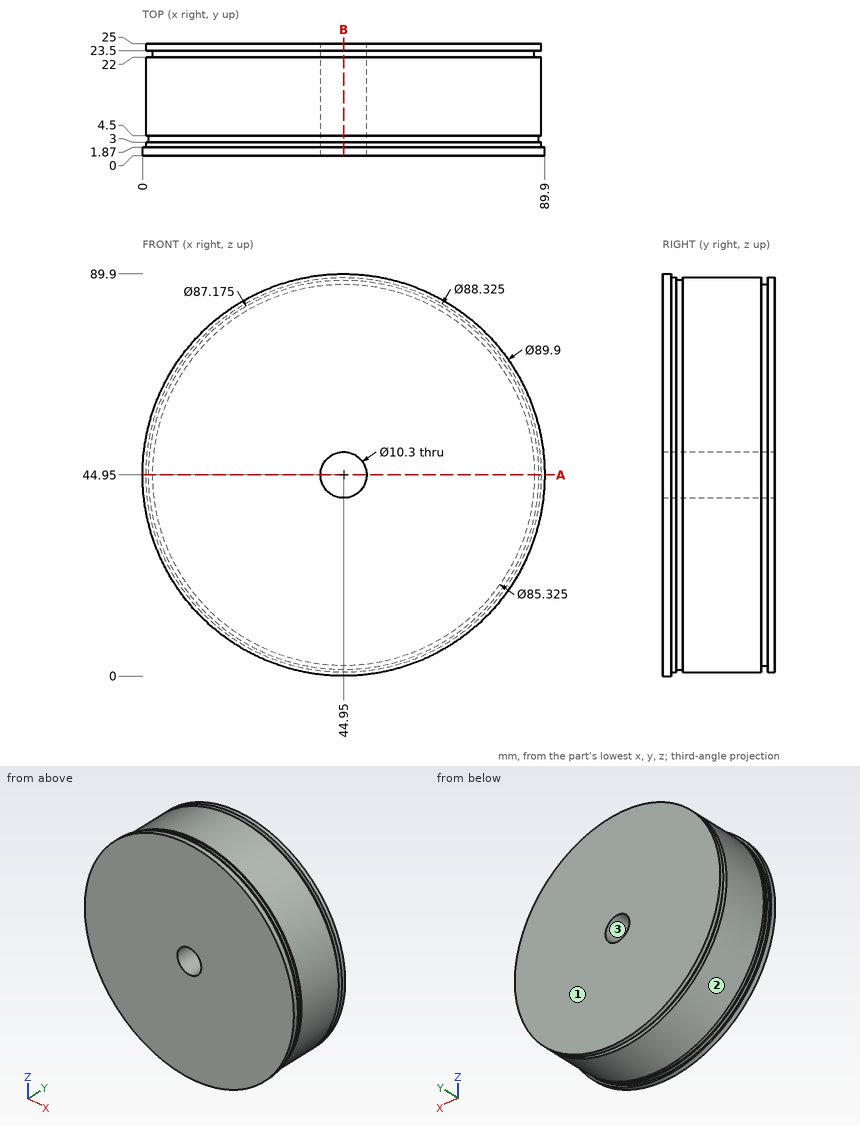
Design review of the part shown in the three views and the two pictorial views. Dimensions are in mm from the part's minimum x, y and z. Round coordinates to 2 decimals unless told otherwise and drop trailing zeros. Order: outer loops, then holes, each group sorted by start corner. A loop starts at its lowest first (then second) coordinate and runs counter-clockwise, first axis right, second up.
(1) Mouldability with a two-part tool opening along X and no side actions: class the marked faces 1, 2 and 3 as released by +X, released by -X, zero draft, split by the parting line, or undercut.
Working result:
face 1: zero draft
face 2: split by the parting line
face 3: undercut
(2) Wall thickness on L1, parallel to Y at x = 7, z = 67; L2, parallel to Z at x = 44.95, y = 17; L3, parallel to X at y = 19.5, z = 38: over which ranges is each line inside the solid? List them lowest first.
Working result:
L1: y = 0 to 3, 4.5 to 22, 23.5 to 25
L2: z = 0.79 to 39.8, 50.1 to 89.11
L3: x = 1.34 to 88.56
(3) Take a section at B-B, the plane x = 44.95. State the section outline as (y, z) points.
Working result:
outline: (0, 0) - (1.87, 0) - (1.87, 0.79) - (3, 0.79) - (3, 1.36) - (4.5, 1.36) - (4.5, 0.79) - (22, 0.79) - (22, 2.29) - (23.5, 2.29) - (23.5, 0.79) - (25, 0.79) - (25, 39.8) - (0, 39.8) - close; (0, 50.1) - (25, 50.1) - (25, 89.11) - (23.5, 89.11) - (23.5, 87.61) - (22, 87.61) - (22, 89.11) - (4.5, 89.11) - (4.5, 88.54) - (3, 88.54) - (3, 89.11) - (1.87, 89.11) - (1.87, 89.9) - (0, 89.9) - close
(4) Take a section at A-A, the plane z = 44.95. State the section outline as (x, y) points.
Working result:
outline: (0, 0) - (39.8, 0) - (39.8, 25) - (0.79, 25) - (0.79, 23.5) - (2.29, 23.5) - (2.29, 22) - (0.79, 22) - (0.79, 4.5) - (1.36, 4.5) - (1.36, 3) - (0.79, 3) - (0.79, 1.87) - (0, 1.87) - close; (50.1, 0) - (89.9, 0) - (89.9, 1.87) - (89.11, 1.87) - (89.11, 3) - (88.54, 3) - (88.54, 4.5) - (89.11, 4.5) - (89.11, 22) - (87.61, 22) - (87.61, 23.5) - (89.11, 23.5) - (89.11, 25) - (50.1, 25) - close
(5) For P1, Ø6, axis at y = 22.5, z = 50.5, coming from the +X side; P2, Ø10, axis at x = 73, y = 14.5, coming from the -Z side; P3, Ø10, axis at y = 3, z = 18, coming from the -X side, all flat-tipped, find the tip position at first contact; note any pin that passes through.
Working result:
P1: stops at x = 89.04
P2: stops at z = 7.28
P3: stops at x = 5.8
